Verification items for the finished model (mm, model axes). A direction names the side the tool comes from. Coordinates: 2 decimals unless noted, no trailing zeros. Order: outer loops, then holes, each group sorted by start corner. A loop starts at its lowest first (then second) coordinate and runs counter-clockwise, first axis right, second up. Notation, with made-up numbers: (51.5, -15.75) -> (85.5, -15.75) arc R30 ccw to (85.5, 15.25) -> close; hole circle Ø9 at (8, 87.5). An arc over 180 degrees is marked (long way). Write item = value, one per line. Start each with the question number.
1. Release check for a two-part mould opening along Y. For faces 1 (the flat face through (20, 16.847, 6)), 2 (the cylindrical face through (12, 31.14, 5.92)), 3 (the flat face through (-6, 7, 0)) record: +Y half, -Y half, draft (parallel to the pull), parting line (faces both ways), or undercut.
2. Thickness scan on line 1 along X through (y, z) = (0, 8.75); line 2 along X through (y, z) = (0, 11.9); line 3 along Y through (x, z) = (-30, 5.75). Record the ranges inside material, lowest first. Write a range as from..to.
3. Cross-section at B-B on y = 0. Record the cut outline in (x, z), plus the area to 3 significant figures.
4. Go/stop test with flat-tipped pins: P1, Ø1.5, axis at y = -4, z = 9, coming from the +X side; P2, Ø2.5, axis at x = -32, z = 6, coming from the -Y side; P3, Ø1.5, axis at y = 3.5, z = 9, coming from the +X side; P4, Ø8, axis at x = -5.74, y = 0, coming from the +Z side. Record where each tip stops, or that it passes through.
5. Set-up check for faces 4 (the flat face through (-32, 0, 10.5)), 5 (the flat face through (21, 0, 1.376)), 6 (the flat face through (-6, 8.793, 2)), 7 (the flat face through (-6, 7.293, 6)): record each of +Z, -Z, +X, -X, +Y, -Y from which the full face is reachable in a straight line by a thin tool's end or side.
6. Cross-section at C-C on y = 18. Record the cut outline in (x, z), plus the area to 3 significant figures.
from build123d import *

# Parameters (mm, degrees)
SKETCH2_R           = 5.075
BOSS_EXTRUDE1_DEPTH = 12
CUT_EXTRUDE1_DEPTH  = 2
SKETCH4_W           = 31.5
SKETCH4_H           = 26.5
CUT_EXTRUDE2_DEPTH  = 2.7
CUT_EXTRUDE3_REACH  = 14
SKETCH5_W           = 18.640557444
SKETCH5_H           = 25
SKETCH6_R           = 11.5
CUT_EXTRUDE4_DEPTH  = 0.5


with BuildPart() as part:
    # Sketch2 → Boss-Extrude1 (new body)
    with BuildSketch(Plane.XY):
        with BuildLine():
            Line((-26.652708458, 24.799544054), (-27.052594325, 20.847218157))
            Line((-27.052594325, 20.847218157), (-35.117996865, 20.847218157))
            Line((-35.117996865, 20.847218157), (-35.117996865, 16.847218157))
            Line((-35.117996865, 16.847218157), (-27.457303732, 16.847218157))
            Line((-27.457303732, 16.847218157), (-28.873786654, 2.847218157))
            Line((-28.873786654, 2.847218157), (-35.117996865, 2.839337807))
            Line((-35.117996865, 2.839337807), (-35.112948764, -1.160662193))
            Line((-35.112948764, -1.160662193), (-28.37093921, -1.152153607))
            Line((-28.37093921, -1.152153607), (-23.24278353, -11.137592085))
            Line((-23.24278353, -11.137592085), (11.75721647, -11.137592085))
            Line((11.75721647, -11.137592085), (16.91451101, -1.09500223))
            Line((16.91451101, -1.09500223), (23.93161739, -1.086146466))
            Line((23.93161739, -1.086146466), (23.92656929, 2.913853534))
            Line((23.92656929, 2.913853534), (17.382313229, 2.905594519))
            Line((17.382313229, 2.905594519), (15.971736672, 16.847218157))
            Line((15.971736672, 16.847218157), (24.207665477, 16.847218157))
            Line((24.207665477, 16.847218157), (24.207665477, 20.847218157))
            Line((24.207665477, 20.847218157), (15.567027266, 20.847218157))
            Line((15.567027266, 20.847218157), (15.167141399, 24.799544054))
            ThreePointArc((15.167141399, 24.799544054), (11.923667067, 31.21134436), (5.217936029, 33.792909804))
            Line((5.217936029, 33.792909804), (-16.703503089, 33.792909804))
            ThreePointArc((-16.703503089, 33.792909804), (-23.409234126, 31.21134436), (-26.652708458, 24.799544054))
        make_face()
        with Locations((-5.74278353, 0)):
            Circle(SKETCH2_R, mode=Mode.SUBTRACT)
    extrude(amount=BOSS_EXTRUDE1_DEPTH)

    # Sketch3 → Cut-Extrude1 (cut)
    with BuildSketch(Plane(origin=(0.001408858, -1.116346991, 0), x_dir=(0.999999204, 0.001262024, 0), z_dir=(0.001262024, -0.999999204, 0))):
        Polygon((-35.114385586, 10.5), (-29.114385586, 10.5), (-29.114385586, 8.5), (-29.114385586, 3.523848556), (-29.114385586, 1.461924081), (-35.114385586, 1.461924081), (-35.114385586, 3.523848556), (-35.114385586, 8.5), align=None)
        Polygon((17.930227589, 10.5), (23.930227589, 10.5), (23.930227589, 8.5), (23.930227589, 3.438075525), (23.930227589, 1.376151049), (17.930227589, 1.376151049), (17.930227589, 3.438075525), (17.930227589, 8.5), align=None)
    extrude(amount=-CUT_EXTRUDE1_DEPTH, mode=Mode.SUBTRACT)

    # Sketch4 → Cut-Extrude2 (cut)
    with BuildSketch(Plane.XY.offset(7)):
        with Locations((-5.74278353, 20.542909804)):
            Rectangle(SKETCH4_W, SKETCH4_H)
    extrude(amount=-CUT_EXTRUDE2_DEPTH, mode=Mode.SUBTRACT)

    # Sketch5 → Cut-Extrude3 (cut, up to next)
    with BuildSketch(Plane(origin=(0, 0, 0), x_dir=(-1, 0, 0), z_dir=(0, 0, -1)), mode=Mode.PRIVATE) as cut_extrude3_sk1:
        with Locations((5.74278353, 21.292909804)):
            Rectangle(SKETCH5_W, SKETCH5_H)
    cut_extrude3_tool1 = extrude(cut_extrude3_sk1.sketch, amount=-CUT_EXTRUDE3_REACH, mode=Mode.PRIVATE) & part.part
    add(cut_extrude3_tool1.solids().sort_by_distance((-5.742784, 21.29291, 0))[0], mode=Mode.SUBTRACT)

    # Sketch6 → Cut-Extrude4 (cut)
    with BuildSketch(Plane.XY.offset(12)):
        with Locations((-5.74278353, 0)):
            Circle(SKETCH6_R)
    extrude(amount=-CUT_EXTRUDE4_DEPTH, mode=Mode.SUBTRACT)


solid = part.part
Worked out:
q1.face_1 = undercut
q1.face_2 = +Y half
q1.face_3 = draft
q2.line_1 = -29.11..-10.82, -0.67..17.93
q2.line_2 = -35.11..-17.24, 5.76..23.93
q2.line_3 = 0.85..2.85, 16.85..20.85
q3.outline = (-35.11, 0) -> (-10.82, 0) -> (-10.82, 11.5) -> (-17.24, 11.5) -> (-17.24, 12) -> (-35.11, 12) -> (-35.11, 10.5) -> (-29.11, 10.5) -> (-29.11, 1.46) -> (-35.11, 1.46) -> close; (-0.67, 0) -> (23.93, 0) -> (23.93, 1.38) -> (17.93, 1.38) -> (17.93, 10.5) -> (23.93, 10.5) -> (23.93, 12) -> (5.76, 12) -> (5.76, 11.5) -> (-0.67, 11.5) -> close
q3.area = 471 mm²
q4.P1 = 15.81
q4.P2 = 0.84
q4.P3 = 23.93
q4.P4 = through
q5.face_4 = -X, -Y
q5.face_5 = +X, -Y
q5.face_6 = -Z, +Y
q5.face_7 = +Y
q6.outline = (-35.12, 0) -> (-15.06, 0) -> (-15.06, 4.3) -> (-21.49, 4.3) -> (-21.49, 7) -> (10.01, 7) -> (10.01, 4.3) -> (3.58, 4.3) -> (3.58, 0) -> (24.21, 0) -> (24.21, 12) -> (-35.12, 12) -> close
q6.area = 547 mm²
